Could you check a few things on this model? Use its own coordinates, in mm. A direction names the side the tool comes from. Give positions to 0.01 mm unless a question says otherwise; leave off trailing zeros. Loops run counter-clockwise (first coordinate to the right, second up) from the corner with the lowest first, then second, coordinate; pieces in that order, holes last. Notation, with made-up numbers: (43, 54) - (51, 54) arc R15 ccw to (51, 81) - close; hole circle Ø4 at (14.5, 56.5). An arc over 180 degrees is marked (long way). Write each question's results on one line, items separated by ' | '. Start each with the question number.
(1) If we mould it in two halves opening along Y, with no side actions, what happens to faces 4 (the face through (-1.341, -205.07, 3.233)), 5 (the face through (-3.3, -200, 2.2)), 6 (the face through (1.05, -212.535, 3.334))? For each: released by +Y, released by -Y, zero draft, split by the parting line, or undercut.
(2) For pin 1 (1.5 mm diameter, centred on x = 2.5, y = 65.5, fed in from +Z); pin 2 (5 mm diameter, centred on y = -45, z = -3, fed in from -X), each with a flat end and sliding along its axis, tell me the tip position at first contact or that it passes through.
(3) I need wall thicknesses on line 1 (Y direction, x = -2.75, z = -1.5); line 2 (Y direction, x = 1, z = -4.5); line 3 (Z direction, x = -4, y = -49). Which ranges of each line are inside material? Lowest first, please.
(4) On a 3-axis mill with a long thin cutter (end or side, diameter ignored), from which of +Z, -Z, +X, -X, +Y, -Y can I reach the whole of each face in a straight line? I mean faces 1 (the face through (0, 210, 0)), 2 (the face through (-1.341, 202.958, 3.233)), 3 (the face through (-2, -215, 2)). Say none if no direction works.
(5) Suppose I cut it at A-A (y = -70.5). Please give me the cut outline in (x, z).
from build123d import *

# Parameters (mm, degrees)
F0_W   = 10
F0_H   = 2.5
F0_W_2 = 0.9
F0_H_2 = 3.25


# Not quite as in the source:
# - a feature names something its author has since deleted; it is built from what else it names


with BuildPart() as f1:
    # F0 (on Right) → F1 (revolve)
    with BuildSketch(Plane.YZ):
        Polygon((200, 3.5), (200, 5), (-200, 5), (-200, 3.5), (-200, 0), (200, 0), align=None)
        Polygon((-200, 0), (-200, 3.5), (-210, 3.5), (-210, 3.48999998), (-210, 0), align=None)
        with Locations((-220, 1.25)):
            Rectangle(F0_W, F0_H)
        Polygon((206, 3.5), (200, 3.5), (200, 0), (206, 0), (206, 3.25), align=None)
        with Locations((206.45, 1.625)):
            Rectangle(F0_W_2, F0_H_2)
        Polygon((206.9, 3.25), (206.9, 0), (210, 0), (210, 3.5), (206.9, 3.5), align=None)
        Polygon((-215, 0), (-210, 0), (-210, 3.48999998), (-215, 3.5), (-215, 2.5), align=None)
    revolve(axis=Axis((0, -7.5, 0), (0, 1, 0)))


solid = f1.part
Output values:
1) face 4: zero draft | face 5: released by -Y | face 6: undercut
2) pin 1: z = 4.68 | pin 2: x = -4.97
3) line 1: -215 to 210 | line 2: -200 to 200 | line 3: -3 to 3
4) face 1: +Z, -Z, +X, -X, +Y | face 2: +Y | face 3: -Y
5) outline: circle Ø10 at (0, 0)
